The model under review builds one solid part; all positions refer to its coordinate system, in mm. Round coordinates to 2 decimals unless told otherwise and drop trailing zeros. Loops run counter-clockwise (first coordinate to the right, second up) from the corner with the lowest first, then second, coordinate; pieces in that order, holes last. Notation, with made-up numbers: (32.25, 72) -> (79.25, 72) arc R17 ccw to (79.25, 89) -> close; hole circle Ø2 at (-39, 58). An arc over 180 degrees is marked (long way). Write each question's results on one line, items separated by ' | '. Start each with the question number.
Item 1: For L1, parallel to X at y = 13.75, z = 1; L2, parallel to Z at x = -11, y = 13.75; L3, parallel to X at y = 4, z = 7.5, list the stretches that pass through material, from the lowest coordinate up. Write a range as from..to.
Item 2: We need section B-B (z = -5.5). Give the boundary of the cut face in (x, y).
Item 3: Mouldability with a two-part tool opening along X and no side actions: class faces 1 (the cylindrical face through (0.07, 7.4, 14.9)), 2 (the cylindrical face through (0, 7.4, 20.5)), 3 (the flat face through (-8, 15, -11)) as pulls with the +X half, pulls with the -X half, needs draft (parallel to the pull), parting line crosses it, or undercut.
Item 4: We need section A-A (y = 6.75). Give the boundary of the cut face in (x, z).
Item 5: We need section D-D (x = 0.5). Give the boundary of the cut face in (y, z), and give its area (3 significant figures).
Item 6: Clearance check with flat-ended pins moving along their axes: pin 1 Ø1.5 at (y, z) = (11, 5) entering from -X; pin 2 Ø2 at (x, y) = (5, 11) entering from -Z; pin 3 Ø1.5 at (y, z) = (2.5, 6) entering from +X; pin 4 Ø3 at (x, z) = (16.5, 0) entering from -Y. State where each tip first meets the part, or that it passes through.
Item 7: We need section C-C (x = -8.5). Give the boundary of the cut face in (y, z).
from build123d import *

# Parameters (mm, degrees)
SKETCH_1_R      = 1.6
SKETCH_1_R_2    = 12.7
EXTRUDE_1_DEPTH = 15


with BuildPart() as part:
    # 草图1 → 凸台-拉伸1 (new body)
    with BuildSketch(Plane(origin=(0, 0, 0), x_dir=(1, 0, 0), z_dir=(0, 1, 0))):
        with BuildLine():
            Line((-3.064936623, 20.269587157), (-20.269587157, 3.064936623))
            ThreePointArc((-20.269587157, 3.064936623), (-20.5, 0), (-20.269587157, -3.064936623))
            Line((-20.269587157, -3.064936623), (-3.064936623, -20.269587157))
            ThreePointArc((-3.064936623, -20.269587157), (0, -20.5), (3.064936623, -20.269587157))
            Line((3.064936623, -20.269587157), (20.269587157, -3.064936623))
            ThreePointArc((20.269587157, -3.064936623), (20.442315631, -1.536792649), (20.5, 0))
            ThreePointArc((20.5, 0), (20.442315631, 1.536792649), (20.269587157, 3.064936623))
            Line((20.269587157, 3.064936623), (3.064936623, 20.269587157))
            ThreePointArc((3.064936623, 20.269587157), (0, 20.5), (-3.064936623, 20.269587157))
        make_face()
        with Locations(Location((-16.5, 0, 0), (0, 0, 270))):
            Circle(SKETCH_1_R, mode=Mode.SUBTRACT)
        with Locations(Location((0, -16.5, 0), (0, 0, 270))):
            Circle(SKETCH_1_R, mode=Mode.SUBTRACT)
        with Locations(Location((0, 0, 0), (0, 0, 270))):
            Circle(SKETCH_1_R_2, mode=Mode.SUBTRACT)
        with Locations(Location((16.5, 0, 0), (0, 0, 270))):
            Circle(SKETCH_1_R, mode=Mode.SUBTRACT)
        with Locations(Location((0, 16.5, 0), (0, 0, 270))):
            Circle(SKETCH_1_R, mode=Mode.SUBTRACT)
    extrude(amount=EXTRUDE_1_DEPTH)


solid = part.part
Here are the results:
1) L1: x = -20.48..-17.75, -15.25..-12.66, 12.66..15.25, 17.75..20.48 | L2: z = -12.33..-6.35, 6.35..12.33 | L3: x = -15.83..-10.25, 10.25..15.83
2) outline: (-17.83, 0) -> (-11.45, 0) -> (-11.45, 15) -> (-17.83, 15) -> close; (11.45, 0) -> (17.83, 0) -> (17.83, 15) -> (11.45, 15) -> close
3) face 1: undercut | face 2: parting line crosses it | face 3: needs draft
4) outline: (-20.27, -3.06) -> (-3.06, -20.27) arc R20.5 ccw to (3.06, -20.27) -> (20.27, -3.06) arc R20.5 ccw to (20.27, 3.06) -> (3.06, 20.27) arc R20.5 ccw to (-3.06, 20.27) -> (-20.27, 3.06) arc R20.5 ccw to start; hole circle Ø3.2 at (-16.5, 0); hole circle Ø25.4 at (0, 0); hole circle Ø3.2 at (0, -16.5); hole circle Ø3.2 at (0, 16.5); hole circle Ø3.2 at (16.5, 0)
5) outline: (0, -20.49) -> (15, -20.49) -> (15, -18.02) -> (0, -18.02) -> close; (0, -14.98) -> (15, -14.98) -> (15, -12.69) -> (0, -12.69) -> close; (0, 12.69) -> (15, 12.69) -> (15, 14.98) -> (0, 14.98) -> close; (0, 18.02) -> (15, 18.02) -> (15, 20.49) -> (0, 20.49) -> close | area: 143 mm2
6) pin 1: stops at x = -19.08 | pin 2: stops at z = -19.33 | pin 3: stops at x = 18.08 | pin 4: passes through
7) outline: (0, -14.83) -> (15, -14.83) -> (15, -9.44) -> (0, -9.44) -> close; (0, 9.44) -> (15, 9.44) -> (15, 14.83) -> (0, 14.83) -> close
